Can you work these out from the drawing? Everything is in mm from the part's minimum corner. Coordinates: 2 decimals unless noted, no trailing zeros. Order: outer loops, then holes, each group sorted by start corner. A loop starts at its lowest first (then second) coordinate and runs counter-clockwise, first axis right, second up. Notation, with made-up numbers: (-10, -34.5) - (30, -34.5) arc R16 cw to (30, -22.5) - close; hole circle Ø6 at (-11, 10.25). An arc over 180 degrees is marked (long way). One line per item, written item: value.
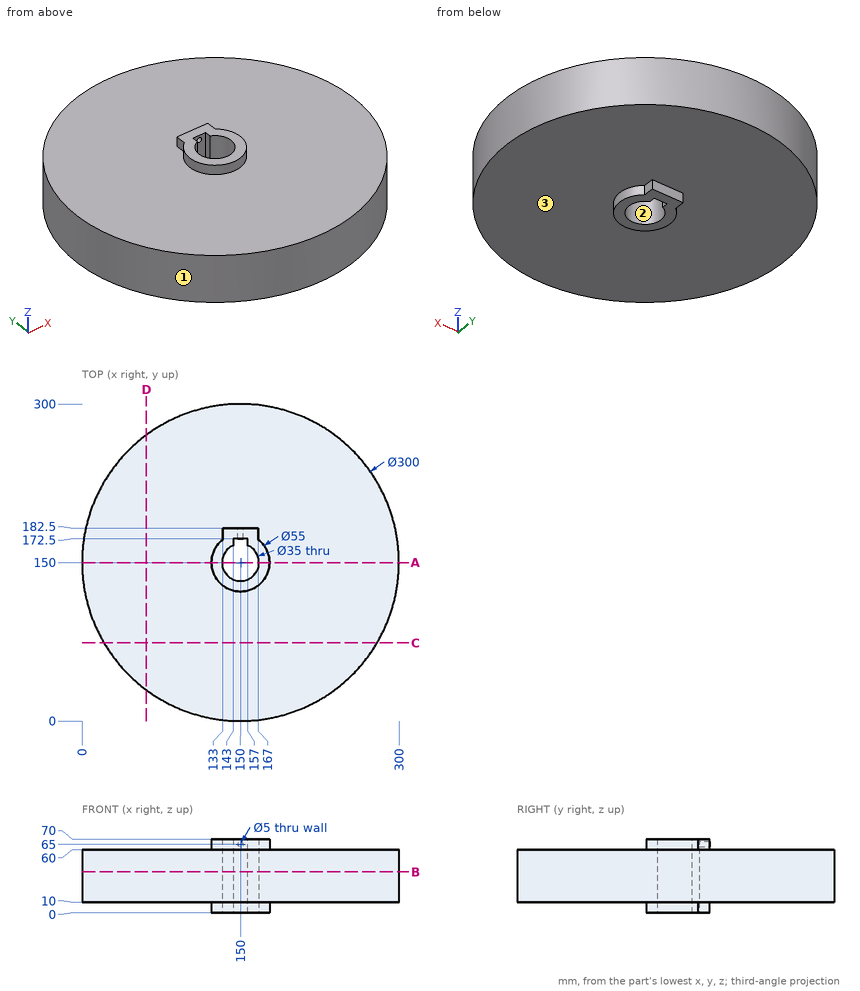
Item 1: Thinking about a two-plate mould opening in Y: for the marked faces 1, 2 and 3, which applies, pulls with the +Y half, pulls with the -Y half, needs draft (parallel to the pull), parting line crosses it, or undercut?
Conclusion:
face 1: parting line crosses it
face 2: undercut
face 3: needs draft
Item 2: I want a section at D-D on x = 61. Please give me the cut outline in (y, z).
Conclusion:
outline: (29.26, 10) - (270.74, 10) - (270.74, 60) - (29.26, 60) - close
Item 3: I'm going to push flat-ended pins straight in: pin 1 Ø3 at (x, z) = (158, 6) entering from +Y; pin 2 Ø12 at (x, y) = (252, 72.5) entering from -Z; pin 3 Ø3 at (x, y) = (139.5, 112) entering from +Z. Where does each tip first touch, or does it pass through?
Conclusion:
pin 1: y = 182.5
pin 2: z = 10
pin 3: z = 60
Item 4: I want a section at B-B on z = 39. Please give me the cut outline in (x, y).
Conclusion:
outline: circle Ø300 at (150, 150); hole (143, 166.04) arc R17.5 ccw (long way) to (157, 166.04) - (157, 172.5) - (143, 172.5) - close
Item 5: I want a section at C-C on y = 74. Please give me the cut outline in (x, z).
Conclusion:
outline: (20.68, 10) - (279.32, 10) - (279.32, 60) - (20.68, 60) - close
Item 6: If I drill on probe 1 along Z at (x, y) = (150, 180.25); probe 2 along Y at (x, z) = (150, 28.5); probe 3 along X at (y, z) = (178.75, 65), over which ranges is the centre line in solid material (lowest first)?
Conclusion:
probe 1: 0 to 62.5, 67.5 to 70
probe 2: 0 to 132.5, 172.5 to 300
probe 3: 133 to 147.5, 152.5 to 167
Item 7: I want a section at A-A on y = 150. Please give me the cut outline in (x, z), then the cut area to 4 significant figures.
Conclusion:
outline: (0, 10) - (122.5, 10) - (122.5, 0) - (132.5, 0) - (132.5, 70) - (122.5, 70) - (122.5, 60) - (0, 60) - close; (167.5, 0) - (177.5, 0) - (177.5, 10) - (300, 10) - (300, 60) - (177.5, 60) - (177.5, 70) - (167.5, 70) - close
area: 13,650 mm²
